Print and shaded views of the part. All mm, measured from the part's lowest x, y and z. A direction names the side the tool comes from. Round coordinates to 2 decimals unless told otherwise and drop trailing zeros. Write each loop counter-clockwise with the first axis right and the second up, starting at its lowest first coordinate (ties: lowest second). Pieces come first, ordered by that corner, then holes. Notation, with made-up numbers: (52.25, 14) -> (110.25, 14) arc R19 cw to (110.25, 45) -> close; hole circle Ø6 at (-28.5, -2.5). An arc over 180 degrees is marked (long way). Use CSV: the item, a comma, the result in double quotes. Start each with the question number.
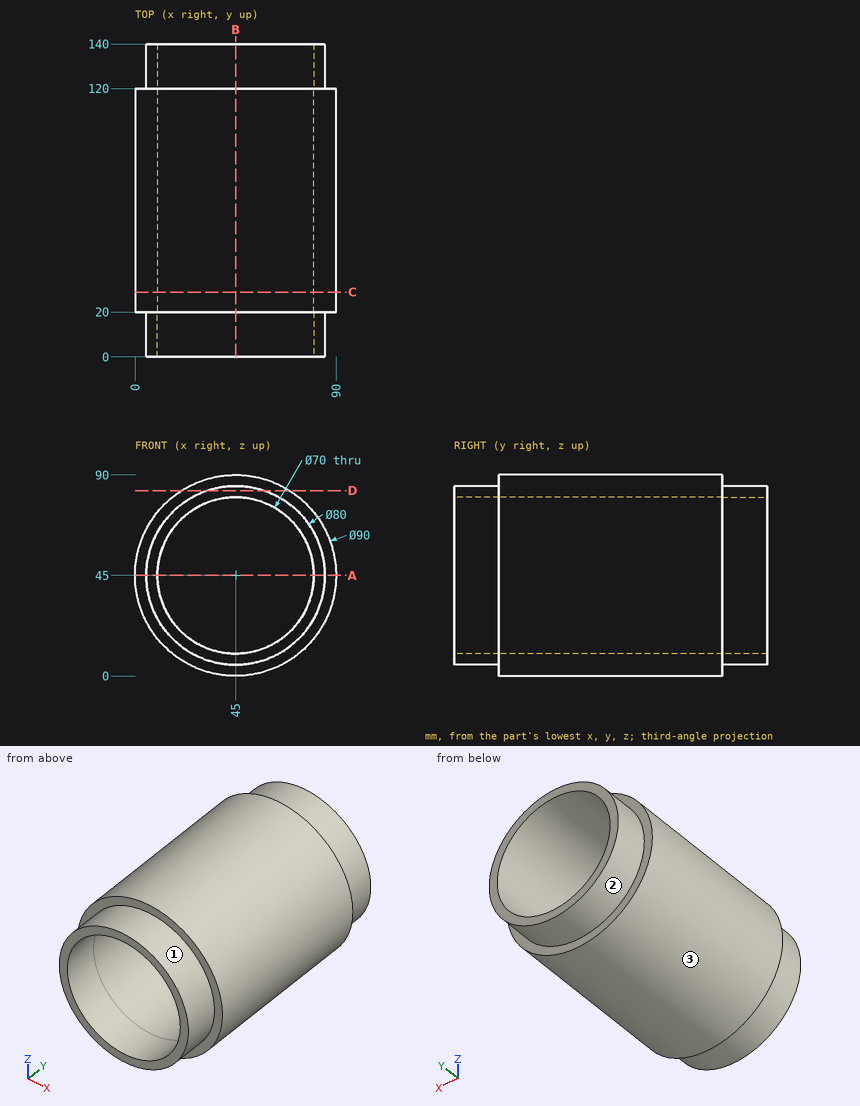
1. Band-saw the part on B-B (x = 45). List the corners of the cut face in (y, z), then the cut area to 3 significant figures.
2. Which spindle directions (+Z, -Z, +X, -X, +Y, -Y) get a long thin tool onto all of the face, cutting with end or side? Do the marked faces 1, 2 and 3. Say none if no direction does.
3. Band-saw the part on D-D (z = 83). List the corners of the cut face in (x, y), then the cut area to 3 significant figures.
4. Band-saw the part on A-A (z = 45). List the corners of the cut face in (x, y), then the cut area to 3 significant figures.
5. Band-saw the part on C-C (y = 29). List the corners of the cut face in (x, z).
6. Drill centre lines: line 1 along Z through (x, y) = (45, 6.75); line 2 along X through (y, z) = (52.5, 45); line 3 along X through (y, z) = (10, 74.5). Where is each one in solid material? Low to high. Write a range as [from, to].
7. Flat gauge pins, fed straight in: pin 1 (1.5 mm diameter, centred on y = 102.5, z = 16.5, fed in from +X); pin 2 (10 mm diameter, centred on x = 52, y = 81, fed in from -Z); pin 3 (8 mm diameter, centred on x = 33.5, y = 23, fed in from -Z); pin 4 (4 mm diameter, centred on x = 15.5, z = 56, fed in from -Y). Where does each tip first touch, or does it go through?
Answers below:
1,outline,"(0, 5) -> (20, 5) -> (20, 0) -> (120, 0) -> (120, 5) -> (140, 5) -> (140, 10) -> (0, 10) -> close; (0, 80) -> (140, 80) -> (140, 85) -> (120, 85) -> (120, 90) -> (20, 90) -> (20, 85) -> (0, 85) -> close"
1,area,"2,400 mm^2"
2,face 1,"-Y"
2,face 2,"+Y"
2,face 3,"+Y, -Y"
3,outline,"(20.9, 20) -> (32.51, 20) -> (32.51, 0) -> (57.49, 0) -> (57.49, 20) -> (69.1, 20) -> (69.1, 120) -> (57.49, 120) -> (57.49, 140) -> (32.51, 140) -> (32.51, 120) -> (20.9, 120) -> close"
3,area,"5,820 mm^2"
4,outline,"(0, 20) -> (5, 20) -> (5, 0) -> (10, 0) -> (10, 140) -> (5, 140) -> (5, 120) -> (0, 120) -> close; (80, 0) -> (85, 0) -> (85, 20) -> (90, 20) -> (90, 120) -> (85, 120) -> (85, 140) -> (80, 140) -> close"
4,area,"2,400 mm^2"
5,outline,"circle Ø90 at (45, 45); hole circle Ø70 at (45, 45)"
6,line 1,"z = [5, 10], [80, 85]"
6,line 2,"x = [0, 10], [80, 90]"
6,line 3,"x = [17.99, 26.17], [63.83, 72.01]"
7,pin 1,"stops at x = 80.43"
7,pin 2,"stops at z = 0.04"
7,pin 3,"stops at z = 0.63"
7,pin 4,"passes through"
